from build123d import *

# Parameters (mm, degrees)
SKETCH1_W           = 12.5
SKETCH1_H           = 13.5
BOSS_EXTRUDE1_DEPTH = 1.5
SKETCH2_W           = 7.5
SKETCH2_H           = 3
BOSS_EXTRUDE2_DEPTH = 2
SKETCH3_R           = 1.5
CUT_EXTRUDE4_DEPTH  = 11.541584321


with BuildPart() as part:
    # Sketch1 → Boss-Extrude1 (new body)
    with BuildSketch(Plane(origin=(0, 0, 0), x_dir=(1, 0, 0), z_dir=(0, 1, 0))):
        Rectangle(SKETCH1_W, SKETCH1_H)
    extrude(amount=BOSS_EXTRUDE1_DEPTH)

    # Sketch2 → Boss-Extrude2 (add)
    with BuildSketch(Plane(origin=(0, 1.5, 0), x_dir=(1, 0, 0), z_dir=(0, 1, 0))):
        with Locations((0, 6.75)):
            Rectangle(SKETCH2_W, SKETCH2_H)
    extrude(amount=BOSS_EXTRUDE2_DEPTH)

    # Sketch3 → Cut-Extrude4 (cut, through all)
    with BuildSketch(Plane(origin=(0, 1.5, 0), x_dir=(1, 0, 0), z_dir=(0, 1, 0))):
        with Locations(Location((-4.5, -1.25, 0), (0, 0, 270))):
            Circle(SKETCH3_R)
        with Locations(Location((4.5, -1.25, 0), (0, 0, 270))):
            Circle(SKETCH3_R)
    extrude(amount=-CUT_EXTRUDE4_DEPTH, mode=Mode.SUBTRACT)


solid = part.part
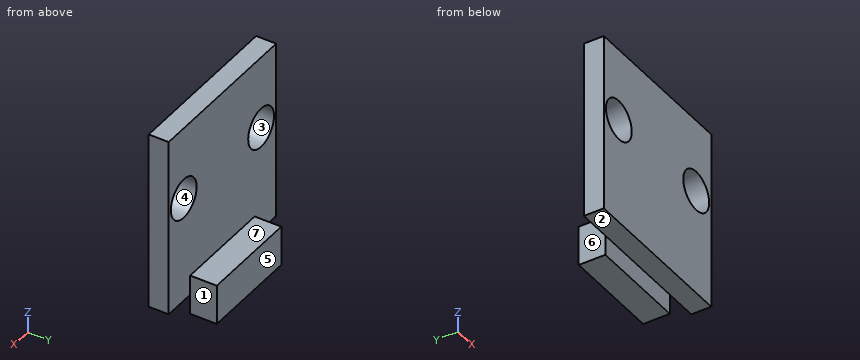
Work out the finished part from the listing and answer in its coordinate system (mm). Face numbers are marked on the shaded views. A direction names the side the tool comes from. Round coordinates to 2 decimals unless told otherwise and drop trailing zeros. Write each loop counter-clockwise with the first axis right and the second up, starting at its lowest first coordinate (ties: lowest second). Pieces come first, ordered by that corner, then holes.
1) A cutting plane is placed at C-C (z = 3.5). Give the vertices of the cut face in (x, y).
2) A cutting plane is placed at A-A (z = 1.25). Give the vertices of the cut face in (x, y), plus the area to 3 significant figures.
3) Given pin 1 Ø1.2 at (x, z) = (-1, -7.5) entering from -Y; pin 2 Ø0.6 at (y, z) = (2.5, -7.5) entering from -X; pin 3 Ø1.5 at (x, y) = (-4, 2.5) entering from +Z, each flat-ended and moving along its own axis, determine where each tip first touches the part or whether it passes through.
4) Straight lines are drawn through the part: line 1 (X direction, y = 0.85, z = 1.25); line 2 (Y direction, x = 0.5, z = -3.75); line 3 (Z direction, x = -0.5, y = 1.05). For each, find the intervals that lie inside material, in ascending order.
5) The mould has two halves that part along Z. Classify the marked faces 1, 2, 3 and 4: pulls with the +Z half, pulls with the -Z half, needs draft (parallel to the pull), parting line crosses it, or undercut.
6) A tool of negligible diameter and unlimited length cuts with its end or side. For the marked faces 5, 6 and 7, from which of +Z, -Z, +X, -X, +Y, -Y can it reach the whole face along a straight path? Write none if from no direction.
7) A cutting plane is placed at D-D (y = 2.9). Give the vertices of the cut face in (x, z).
8) A cutting plane is placed at B-B (x = 4.5). Give the vertices of the cut face in (y, z).
Completed:
1. outline: (-6.25, 0) - (6.25, 0) - (6.25, 1.5) - (-6.25, 1.5) - close
2. outline: (-6.25, 0) - (-6, 0) - (-6, 1.5) - (-6.25, 1.5) - close; (-3, 0) - (3, 0) - (3, 1.5) - (-3, 1.5) - close; (6, 0) - (6.25, 0) - (6.25, 1.5) - (6, 1.5) - close
2. area: 9.75 mm2
3. pin 1: stops at y = 1.5
3. pin 2: stops at x = -3.75
3. pin 3: stops at z = -5.25
4. line 1: x = -6.25 to -6, -3 to 3, 6 to 6.25
4. line 2: y = 0 to 1.5
4. line 3: z = -6.75 to 6.75
5. face 1: needs draft
5. face 2: pulls with the -Z half
5. face 3: undercut
5. face 4: undercut
6. face 5: +Z, -Z, +X, -X, +Y
6. face 6: +Z, -Z, -X, +Y
6. face 7: +Z, +X, -X, +Y
7. outline: (-3.75, -8.25) - (3.75, -8.25) - (3.75, -5.25) - (-3.75, -5.25) - close
8. outline: (0, -6.75) - (1.5, -6.75) - (1.5, -0.25) - (0, -0.25) - close; (0, 2.75) - (1.5, 2.75) - (1.5, 6.75) - (0, 6.75) - close
